Here's how the part is built. I have some questions about the finished solid (model axes, mm). A direction names the side the tool comes from. Give positions to 0.01 mm unless a question says otherwise; leave off trailing zeros. Loops run counter-clockwise (first coordinate to the right, second up) from the corner with the lowest first, then second, coordinate; pieces in that order, holes last. Notation, with made-up numbers: (-25.5, 12.5) - (18.5, 12.5) arc R18 ccw to (18.5, 19.5) - close; hole circle Ø8 at (21, -14). An arc over 180 degrees is marked (long way). Use a Markdown table: item, result.
from build123d import *

# Parameters (mm, degrees)
SKETCH_1_W          = 25
SKETCH_1_H          = 40
EXTRUDE_1_DEPTH     = 4
SKETCH_2_R          = 2
CUT_EXTRUDE_1_DEPTH = 10
FILLET_1_R          = 2
SKETCH_3_W          = 16
SKETCH_3_H          = 24
CUT_EXTRUDE_2_DEPTH = 10
FILLET_2_R          = 2


with BuildPart() as part:
    # 草图1 → 凸台-拉伸1 (new body)
    with BuildSketch(Plane.XY):
        Rectangle(SKETCH_1_W, SKETCH_1_H)
    extrude(amount=EXTRUDE_1_DEPTH)

    # 草图2 → 切除-拉伸1 (cut)
    with BuildSketch(Plane.XY.offset(4)):
        with Locations((0, 15)):
            Circle(SKETCH_2_R)
        with Locations((0, -15)):
            Circle(SKETCH_2_R)
    extrude(amount=-CUT_EXTRUDE_1_DEPTH, mode=Mode.SUBTRACT)

    # 圆角1
    fillet_1_edges = [part.edges().sort_by_distance(p)[0] for p in [
        (12.5, -20, 2),
        (-12.5, -20, 2),
        (-12.5, 20, 2),
        (12.5, 20, 2),
    ]]
    fillet(fillet_1_edges, radius=FILLET_1_R)

    # 草图3 → 切除-拉伸2 (cut)
    with BuildSketch(Plane.XY.offset(4)):
        Rectangle(SKETCH_3_W, SKETCH_3_H)
    extrude(amount=-CUT_EXTRUDE_2_DEPTH, mode=Mode.SUBTRACT)

    # 圆角2
    fillet_2_edges = [part.edges().sort_by_distance(p)[0] for p in [
        (8, 12, 2),
        (8, -12, 2),
        (-8, -12, 2),
        (-8, 12, 2),
    ]]
    fillet(fillet_2_edges, radius=FILLET_2_R)


solid = part.part
(1) If I drill on line 1 (Y direction, x = 0, z = 0.55); line 2 (Y direction, x = 2.5, z = 3); line 3 (X direction, y = 1.5, z = 1.5), over which ranges is the centre line in solid material (lowest first)?
A:
| item | result |
|---|---|
| line 1 | -20 to -17, -13 to -12, 12 to 13, 17 to 20 |
| line 2 | -20 to -12, 12 to 20 |
| line 3 | -12.5 to -8, 8 to 12.5 |
(2) We'd pull the mould along Y, two halves only. Please class faces 3 (the face through (0, 20, 2)), 4 (the face through (-8, 0, 2)), 5 (the face through (-9, 0, 0)), 6 (the face through (0, -20, 2)): pulls with the +Y half, pulls with the -Y half, needs draft (parallel to the pull), parting line crosses it, or undercut.
A:
| item | result |
|---|---|
| face 3 | pulls with the +Y half |
| face 4 | undercut |
| face 5 | needs draft |
| face 6 | pulls with the -Y half |
(3) Suppose I cut it at B-B on y = 15. Write out the boundary of the cut face in (x, z), plus the area to 3 significant figures.
A:
| item | result |
|---|---|
| outline | (-12.5, 0) - (-2, 0) - (-2, 4) - (-12.5, 4) - close; (2, 0) - (12.5, 0) - (12.5, 4) - (2, 4) - close |
| area | 84.0 mm2 |
(4) Suppose I cut it at D-D on z = 2.85. Write out the boundary of the cut face in (x, y).
A:
| item | result |
|---|---|
| outline | (-12.5, -18) arc R2 ccw to (-10.5, -20) - (10.5, -20) arc R2 ccw to (12.5, -18) - (12.5, 18) arc R2 ccw to (10.5, 20) - (-10.5, 20) arc R2 ccw to (-12.5, 18) - close; hole (-8, -10) arc R2 ccw to (-6, -12) - (6, -12) arc R2 ccw to (8, -10) - (8, 10) arc R2 ccw to (6, 12) - (-6, 12) arc R2 ccw to (-8, 10) - close; hole circle Ø4 at (0, -15); hole circle Ø4 at (0, 15) |
(5) On a 3-axis mill with a long thin cutter (end or side, diameter ignored), from which of +Z, -Z, +X, -X, +Y, -Y can I reach the whole of each face in a straight line? I mean faces 1 (the face through (-9, 0, 4)), 2 (the face through (-7.4, -11.43, 1.97)). Say none if no direction works.
A:
| item | result |
|---|---|
| face 1 | +Z, +X, -X, +Y, -Y |
| face 2 | +Z, -Z |
(6) Suppose I cut it at C-C on x = 0. Write out the boundary of the cut face in (y, z), plus the area to 3 significant figures.
A:
| item | result |
|---|---|
| outline | (-20, 0) - (-17, 0) - (-17, 4) - (-20, 4) - close; (-13, 0) - (-12, 0) - (-12, 4) - (-13, 4) - close; (12, 0) - (13, 0) - (13, 4) - (12, 4) - close; (17, 0) - (20, 0) - (20, 4) - (17, 4) - close |
| area | 32.0 mm2 |
(7) Suppose I cut it at A-A on x = 3.75. Write out the boundary of the cut face in (y, z), plus the area to 3 significant figures.
A:
| item | result |
|---|---|
| outline | (-20, 0) - (-12, 0) - (-12, 4) - (-20, 4) - close; (12, 0) - (20, 0) - (20, 4) - (12, 4) - close |
| area | 64.0 mm2 |
